Here's how the part is built. I have some questions about the finished solid (model axes, mm). Coordinates: 2 decimals unless noted, no trailing zeros.
(1) For pin 1 Ø1.6 at (y, z) = (-31.5, 1.5) entering from -X; pin 2 Ø1.5 at (x, z) = (67.5, 2) entering from -Y; pin 3 Ø0.8 at (x, z) = (-74.5, 1) entering from -Y, each with a flat end and sliding along its axis, tell me the tip position at first contact or that it passes through.
(2) Please list where these lines run through material, in increasing order: probe 1 along X at (y, z) = (-35.5, 1.8); probe 2 along X at (y, z) = (-40, 2.35); probe 3 along X at (y, z) = (-9, 0.2).
(3) Thinking about a two-plate mould opening in X: for faces 1 (the flat face through (-27, -7, 3.175)), 2 (the cylindrical face through (-51.99, -29.52, 1.61)), which applies, released by +X, released by -X, zero draft, split by the parting line, or undercut?
```python
from build123d import *

# Parameters (mm, degrees)
BOSS_EXTRUDE1_DEPTH = 3.175
SKETCH3_W           = 10
SKETCH3_H           = 6.35
BOSS_EXTRUDE2_DEPTH = 3.175
SKETCH4_R           = 5
CUT_EXTRUDE1_DEPTH  = 114.626458313
CUT_EXTRUDE2_DEPTH  = 114.626458313


with BuildPart() as part:
    # Sketch2 → Boss-Extrude1 (new body)
    with BuildSketch(Plane.XY):
        with BuildLine():
            Line((-100.609869354, -40.604219784), (-21.744841678, -40.604219784))
            add(Edge.make_bspline(
                [(89.238978774, 52.511300132), (2.91962202, 37.989392405), (-21.744841678, -40.604219784)],
                knots=[0, 0, 0, 1, 1, 1], degree=2))
            add(Edge.make_bspline(
                [(89.238978774, 52.511300132), (45.213595461, 54.960877806), (4.522727388, 34.592562225), (-32.259998233, 12.458533919)],
                knots=[0, 0, 0, 0, 1, 1, 1, 1], degree=3))
            add(Edge.make_bspline(
                [(-32.259998233, 12.458533919), (-77.388125592, 3.705886884), (-100.609869354, -40.604219784)],
                knots=[0, 0, 0, 1, 1, 1], degree=2))
        make_face()
    extrude(amount=BOSS_EXTRUDE1_DEPTH)

    # Sketch3 → Boss-Extrude2 (add)
    with BuildSketch(Plane.XY.offset(3.175)):
        with Locations((-85.609869354, -43.779219784)):
            Rectangle(SKETCH3_W, SKETCH3_H)
        with Locations((-50.609869354, -43.779219784)):
            Rectangle(SKETCH3_W, SKETCH3_H)
    extrude(amount=-BOSS_EXTRUDE2_DEPTH)

    # Sketch4 → Cut-Extrude1 (cut, through all)
    with BuildSketch(Plane.XY.offset(3.175)):
        with Locations((-56.609869354, -27.604219784)):
            Circle(SKETCH4_R)
    extrude(amount=-CUT_EXTRUDE1_DEPTH, mode=Mode.SUBTRACT)

    # Sketch5 → Cut-Extrude2 (cut, through all)
    with BuildSketch(Plane.XY.offset(3.175)):
        Polygon((-74.109869354, -37.604219784), (-74.109869354, -40.604219784), (-71.109869354, -40.604219784), (-71.109869354, -37.604219784), (-69.559869354, -37.604219784), (-69.559869354, -35.204219784), (-71.109869354, -35.204219784), (-71.109869354, -28.954219784), (-74.109869354, -28.954219784), (-74.109869354, -35.204219784), (-75.659869354, -35.204219784), (-75.659869354, -37.604219784), align=None)
    extrude(amount=-CUT_EXTRUDE2_DEPTH, mode=Mode.SUBTRACT)


solid = part.part
```
Recorded:
1. pin 1: stops at x = -95.87
1. pin 2: stops at y = 47.33
1. pin 3: stops at y = -40.6
2. probe 1: x = -97.79 to -75.66, -69.56 to -20.05
2. probe 2: x = -100.29 to -74.11, -71.11 to -21.55
2. probe 3: x = -76.51 to -7.83
3. face 1: zero draft
3. face 2: undercut
